Could you check a few things on this model? Use its own coordinates, in mm. Coordinates: 2 decimals unless noted, no trailing zeros. Loops run counter-clockwise (first coordinate to the right, second up) from the corner with the lowest first, then second, coordinate; pieces in that order, holes last.
1) Imagine slicing it at A-A on y = 10.5. Please give me the cut outline in (x, z).
2) Imagine slicing it at B-B on z = -56.5. Please give me the cut outline in (x, y), plus the area to 3 significant figures.
3) If I drill on line 1 along X through (y, z) = (17, -49.5); line 2 along X through (y, z) = (13, -48); line 3 along Z through (x, y) = (101, 10.25), over which ranges is the centre line in solid material (lowest first)?
4) Imagine slicing it at D-D on z = -13. Please give me the cut outline in (x, y).
5) Will these pins go through, and if not, where does the flat tip stop? P1, Ø10, axis at y = 6.5, z = -62.5, coming from the -X side; P2, Ø1.5, axis at y = 6.5, z = -41, coming from the +X side; P3, Ø10, axis at x = 98, z = -44.5, coming from the -Y side.
6) Imagine slicing it at C-C on x = 100. Please give me the cut outline in (y, z), plus the area to 3 significant figures.
```python
from build123d import *

# Parameters (mm, degrees)
BOSS_EXTRUDE1_DEPTH = 19
CUT_EXTRUDE1_DEPTH  = 70


with BuildPart() as part:
    # Sketch1 → Boss-Extrude1 (new body)
    with BuildSketch(Plane(origin=(0, 0, 0), x_dir=(1, 0, 0), z_dir=(0, 1, 0))):
        with BuildLine():
            Line((0, 0), (90, 0))
            ThreePointArc((90, 0), (98.219216869, 1.986116209), (104.624620421, 7.506169549))
            ThreePointArc((104.624620421, 7.506169549), (110, 35), (104.624620421, 62.493830451))
            ThreePointArc((104.624620421, 62.493830451), (98.219216869, 68.013883791), (90, 70))
            Line((90, 70), (0, 70))
            Line((0, 70), (0, 0))
        make_face()
    extrude(amount=BOSS_EXTRUDE1_DEPTH)

    # Sketch3 → Cut-Extrude1 (cut)
    with BuildSketch(Plane.XY):
        Polygon((110, 5), (80, 0), (110, 0), align=None)
    extrude(amount=-CUT_EXTRUDE1_DEPTH, mode=Mode.SUBTRACT)


solid = part.part
```
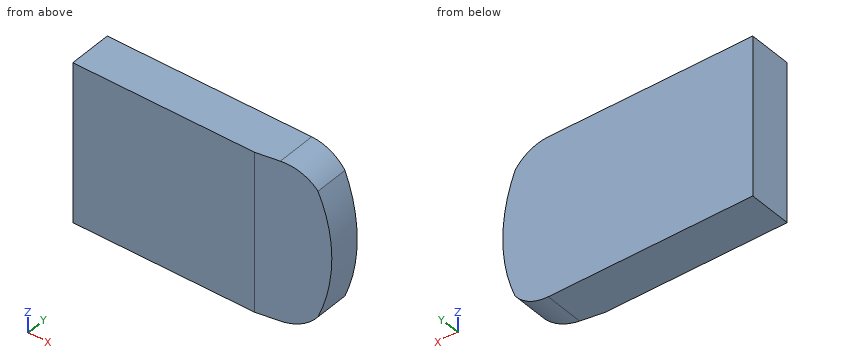
Filled in:
1. outline: (0, -70) - (90, -70) arc R18 ccw to (104.62, -62.49) arc R73 ccw to (104.62, -7.51) arc R18 ccw to (90, 0) - (0, 0) - close
2. outline: (0, 0) - (80, 0) - (106.76, 4.46) - (106.76, 19) - (0, 19) - close
2. area: 1,970 mm2
3. line 1: x = 0 to 108.55
3. line 2: x = 0 to 108.83
3. line 3: z = -66.25 to -3.75
4. outline: (0, 0) - (80, 0) - (106.61, 4.43) - (106.61, 19) - (0, 19) - close
5. P1: stops at x = 0
5. P2: stops at x = 109.81
5. P3: stops at y = 2.17
6. outline: (3.33, -66.97) - (19, -66.97) - (19, -3.03) - (3.33, -3.03) - close
6. area: 1,000 mm2
